The model under review builds one solid part; all positions refer to its coordinate system, in mm. Face numbers are marked on the shaded views. A direction names the side the tool comes from. Round coordinates to 2 decimals unless told otherwise and drop trailing zeros. Order: outer loops, then holes, each group sorted by start corner. A loop starts at its lowest first (then second) coordinate and runs counter-clockwise, first axis right, second up. Notation, with made-up numbers: M 83,13.5 L 91,13.5 A34 ccw 91,45.5 Z; hole C 40.5,-40 d7. An arc over 180 degrees is marked long. Answer as a JSON object with one key per item and string values. Group by question number.
1) Consider section A-A, the plane z = 66.75. Write out the cut boundary in (x, y).
2) Insertion check: pin 1 Ø4 at (x, z) = (1.5, 67.5) entering from -Y; pin 2 Ø1.2 at (x, y) = (1, -16.5) entering from +Z; pin 3 Ø1.1 at (x, z) = (0, 53) entering from +Y; pin 4 Ø2.5 at (x, z) = (-8.75, 32.4) entering from +Y. Each pin has a flat end and moves straight along its axis. Give the tip position at first contact, or say it passes through.
3) Consider section D-D, the plane y = 15. Write out the cut boundary in (x, z), then the cut area to 3 significant figures.
4) To check wall thickness, follow line 1 (X direction, y = -5, z = 32); line 2 (Z direction, x = 0, y = 15); line 3 (Z direction, x = 8.75, y = -5.5). State the ranges of each line that lie inside material, in increasing order.
5) Consider section C-C, the plane x = 4. Write out the cut boundary in (y, z), then the cut area to 3 significant figures.
6) For the marked faces 1 and 2, list the 3-axis set-ups (+Z, -Z, +X, -X, +Y, -Y) from which the entire face can be reached by the end or side of a thin tool; tool diameter is ignored.
7) Consider section B-B, the plane y = -6. Write out the cut boundary in (x, z), then the cut area to 3 significant figures.
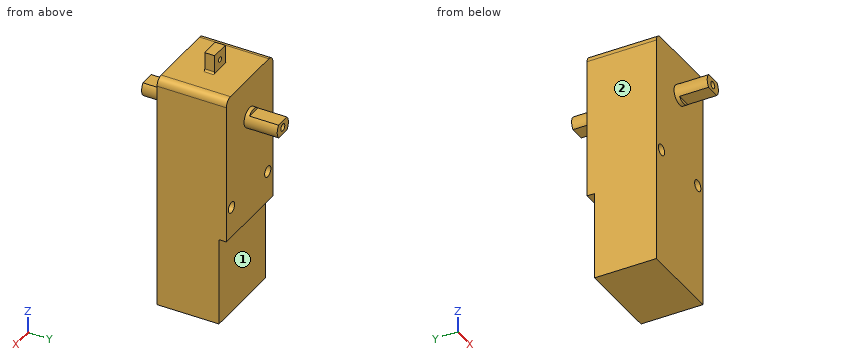
Solid Edge part; units mm, degrees
sketch "Sketch1" plane through (0, 0, 0) normal (0, 0, 1) x (1, 0, 0)
  line L0 (-11.25, -9.4) -> (11.25, -9.4)
  line L1 (11.25, -9.4) -> (11.25, 9.4)
  line L2 (11.25, 9.4) -> (-11.25, 9.4)
  line L3 (-11.25, 9.4) -> (-11.25, -9.4)
  dimension "D1" = 11.25
  dimension "D2" = 11.25
extrude "Ajout_matière_1" add sketch "Sketch1" along normal blind 64.2
sketch "Sketch2" plane through (0, -9.4, 32.1) normal (0, -1, 0) x (1, 0, 0)
  circle A0 centre (0, 20.9) radius 2.7
extrude "Ajout_matière_2" add sketch "Sketch2" along normal blind 9
sketch "Sketch3" plane through (0, -18.4, 53) normal (0, -1, 0) x (1, 0, 0)
  circle A0 centre (0, 0) radius 0.95
extrude "Cutout1" cut sketch "Sketch3" against normal up to vertex (9 mm away)
sketch "Sketch4" plane through (0, -18.4, 53) normal (0, -1, 0) x (1, 0, 0)
  line L0 (2.0125, 1.8) -> (-2.0125, 1.8)
  arc A0 (-2.0125, 1.8) -> (2.0125, 1.8) centre (0, 0) cw
  line L1 (-2.0125, -1.8) -> (2.0125, -1.8)
  arc A1 (-2.0125, -1.8) -> (2.0125, -1.8) centre (0, 0) ccw
  dimension "D1" = 2.0125
  dimension "D2" = 2.0125
extrude "Enlèvement_matière_2" cut sketch "Sketch4" against normal blind 7.9
sketch "Sketch5" plane through (0, 0, 64.2) normal (0, 0, 1) x (0, 1, 0)
  line L0 (-1.35, -2.55) -> (1.35, -2.55)
  line L1 (1.35, -2.55) -> (1.35, 2.55)
  line L2 (1.35, 2.55) -> (-1.35, 2.55)
  line L3 (-1.35, 2.55) -> (-1.35, -2.55)
  dimension "D1" = 1.35
  dimension "D2" = 1.35
extrude "Ajout_matière_3" add sketch "Sketch5" along normal blind 5.1
sketch "Sketch6" plane through (0, -1.35, 65.4) normal (0, -1, 0) x (1, 0, 0)
  circle A0 centre (0, 1.35) radius 0.7
extrude "Cutout2" cut sketch "Sketch6" against normal through all
sketch "Sketch7" plane through (0, -9.4, 32.1) normal (0, -1, 0) x (1, 0, 0)
  circle A0 centre (8.75, 0.3) radius 1.5
extrude "Cutout3" cut sketch "Sketch7" against normal through all
mirror "Mirror1" about plane through (0, 0, 0) normal (1, 0, 0) of "Cutout3"
mirror "Mirror2" about plane through (0, 0, 0) normal (0, -1, 0) of "Ajout_matière_2", "Cutout1", "Enlèvement_matière_2"
fillet "Congé_1" radius 2 2 edges at (11.25, 0, 64.2) (-11.25, 0, 64.2)
fillet "Congé_2" radius 0.5 2 edges at (-2.55, 0, 64.2) (2.55, 0, 64.2)
sketch "Sketch8" plane through (0, 9.4, 32.1) normal (0, 1, 0) x (-1, 0, 0)
  line L0 (-11.25, -32.1) -> (11.25, -32.1)
  line L1 (11.25, -32.1) -> (11.25, -8.1)
  line L2 (11.25, -8.1) -> (-11.25, -8.1)
  line L3 (-11.25, -8.1) -> (-11.25, -32.1)
  dimension "D1" = 11.25
extrude "Enlèvement_matière_8" cut sketch "Sketch8" against normal blind 2
properties material "Acier S235"
Results list:
{
 "1": {"outline": "M -2.55,-1.35 L -0.7,-1.35 L -0.7,1.35 L -2.55,1.35 Z; M 0.7,-1.35 L 2.55,-1.35 L 2.55,1.35 L 0.7,1.35 Z"},
 "2": {"pin 1": "y = -1.35", "pin 2": "z = 54.8", "pin 3": "y = 9.4", "pin 4": "through"},
 "3": {"outline": "M -2.01,51.2 L 2.01,51.2 A2.7 ccw 2.01,54.8 L -2.01,54.8 A2.7 ccw Z; hole C 0,53 d1.9", "area": "15.0 mm^2"},
 "4": {"line 1": "-11.25 to -10.2, -7.3 to 7.3, 10.2 to 11.25", "line 2": "51.2 to 52.05, 53.95 to 54.8", "line 3": "0 to 30.9, 33.9 to 64.2"},
 "5": {"outline": "M -9.4,0 L 7.4,0 L 7.4,24 L 9.4,24 L 9.4,64.2 L -9.4,64.2 Z", "area": "1,160 mm^2"},
 "6": {"face 1": "-Z, +X, -X, +Y", "face 2": "+Z, -Z, -X, +Y, -Y"},
 "7": {"outline": "M -11.25,0 L 11.25,0 L 11.25,62.2 A2 ccw 9.25,64.2 L -9.25,64.2 A2 ccw -11.25,62.2 Z; hole C -8.75,32.4 d3; hole C 8.75,32.4 d3", "area": "1,430 mm^2"}
}
